Print and shaded views of the part. All mm, measured from the part's lowest x, y and z. A direction names the side the tool comes from. Coordinates: 2 decimals unless noted, no trailing zeros. Order: outer loops, then holes, each group sorted by start corner. A loop starts at its lowest first (then second) coordinate and runs counter-clockwise, first axis right, second up. Notation, with made-up numbers: (34, 41) -> (92, 41) arc R9 ccw to (92, 55) -> close; hole circle Ø5 at (10.25, -31.5). An arc over 180 degrees is marked (long way). Write item = value, one per line. Start each with the question number.
Q1. Cut at B-B, the plane z = 3. List the corners of the cut face in (x, y).
Q2. 3-axis set-ups, long thin cutter, end or side, ignore diameter. For the marked faces 5 and 6: which of +Z, -Z, +X, -X, +Y, -Y reach the whole face in a straight line?
Q3. Flat gauge pins, fed straight in: pin 1 (2 mm diameter, centred on y = 26, z = 15, fed in from -X); pin 2 (10 mm diameter, centred on y = 26.5, z = 10.5, fed in from +X); pin 3 (6.5 mm diameter, centred on x = 22, y = 14.5, fed in from +Z); pin 4 (1.5 mm diameter, centred on x = 24, z = 9, fed in from +Y). Where does each tip first touch, or does it go through?
Q4. Cut at A-A, the plane y = 17.5. List the corners of the cut face in (x, z), plus the area to 3 significant figures.
Q5. Wall check: line 1 (Y direction, x = 17.5, z = 13.4); line 2 (X direction, y = 9, z = 10.75); line 3 (Y direction, x = 17.5, z = 16.2). Give the ranges that are in metal, low to high. Write a range as from..to.
Q6. Mould opens along Z. For the marked faces 1, 2, 3 and 4 say: +Z half, -Z half, draft (parallel to the pull), parting line (faces both ways), or undercut.
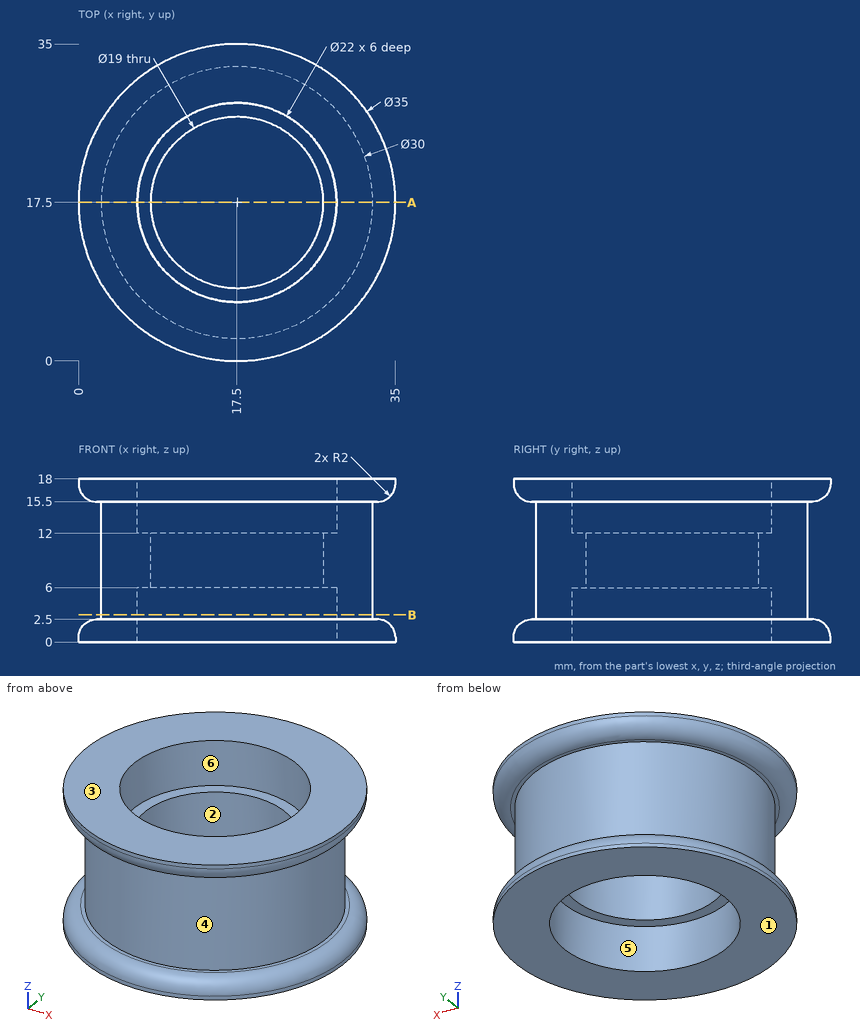
Here are the results:
q1.outline = circle Ø30 at (17.5, 17.5); hole circle Ø22 at (17.5, 17.5)
q2.face_5 = -Z
q2.face_6 = +Z
q3.pin_1 = 2.87
q3.pin_2 = 31.96
q3.pin_3 = through
q3.pin_4 = 31.35
q4.outline = (0, 0) -> (6.5, 0) -> (6.5, 6) -> (8, 6) -> (8, 12) -> (6.5, 12) -> (6.5, 18) -> (0, 18) -> (0, 17.5) arc R2 ccw to (2, 15.5) -> (2.5, 15.5) -> (2.5, 2.5) -> (2, 2.5) arc R2 ccw to (0, 0.5) -> close; (27, 6) -> (28.5, 6) -> (28.5, 0) -> (35, 0) -> (35, 0.5) arc R2 ccw to (33, 2.5) -> (32.5, 2.5) -> (32.5, 15.5) -> (33, 15.5) arc R2 ccw to (35, 17.5) -> (35, 18) -> (28.5, 18) -> (28.5, 12) -> (27, 12) -> close
q4.area = 184 mm²
q5.line_1 = 2.5..6.5, 28.5..32.5
q5.line_2 = 5.14..13.26, 21.74..29.86
q5.line_3 = 0.48..6.5, 28.5..34.52
q6.face_1 = -Z half
q6.face_2 = draft
q6.face_3 = +Z half
q6.face_4 = undercut
